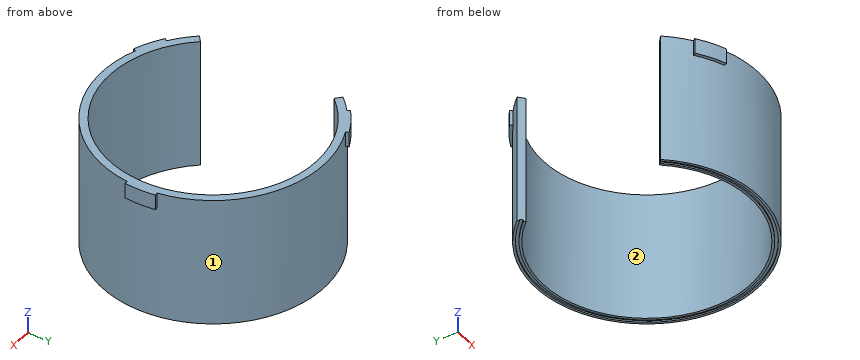
```python
from build123d import *

# Parameters (mm, degrees)
F3_DEPTH = 10
F5_DEPTH = 85


with BuildPart() as f1:
    # F0 (on Front) → F1 (revolve)
    with BuildSketch(Plane.XZ):
        Polygon((-68, 0), (-73, 0), (-73, -85), (-71.5, -85), (-71.5, -84), (-69.5, -84), (-69.5, -85), (-68, -85), align=None)
    revolve(axis=Axis((0, 0, -12.456594), (0, 0, -1)))

    # F2 (on face) → F3 (join)
    with BuildSketch(Plane.XY):
        with BuildLine():
            Line((-25.651511, -70.476947), (-24.96747, -68.597561))
            ThreePointArc((-24.96747, -68.597561), (-33.707649, -64.751791), (-41.87108, -59.798099))
            Line((-41.87108, -59.798099), (-43.018233, -61.436403))
            ThreePointArc((-43.018233, -61.436403), (-34.631146, -66.525812), (-25.651511, -70.476947))
        make_face()
        with BuildLine():
            Line((73.860581, 13.023613), (71.890966, 12.676317))
            ThreePointArc((71.890966, 12.676317), (72.93052, 3.184215), (72.722213, -6.362369))
            Line((72.722213, -6.362369), (74.714602, -6.536681))
            ThreePointArc((74.714602, -6.536681), (74.928617, 3.271454), (73.860581, 13.023613))
        make_face()
        with BuildLine():
            Line((-48.209071, 57.453333), (-46.923496, 55.921244))
            ThreePointArc((-46.923496, 55.921244), (-39.222871, 61.567576), (-30.851133, 66.160468))
            Line((-30.851133, 66.160468), (-31.69637, 67.973084))
            ThreePointArc((-31.69637, 67.973084), (-40.297471, 63.254358), (-48.209071, 57.453333))
        make_face()
    extrude(amount=-F3_DEPTH)

    # F4 (on face) → F5 (cut, through all)
    with BuildSketch(Plane.XY):
        with BuildLine():
            ThreePointArc((-55.509635, 47.409708), (-73, 0), (-55.509635, -47.409708))
            Line((-55.509635, -47.409708), (-51.707606, -44.162467))
            ThreePointArc((-51.707606, -44.162467), (-68, 0), (-51.707606, 44.162467))
            Line((-51.707606, 44.162467), (-55.509635, 47.409708))
        make_face()
    extrude(amount=-F5_DEPTH, mode=Mode.SUBTRACT)


solid = f1.part
```
For this review, take the finished solid that the model builds, in its own axes (mm). Face numbers are marked on the shaded views. A direction names the side the tool comes from. Give positions to 0.01 mm unless a question says otherwise; leave off trailing zeros. Write each loop counter-clockwise with the first axis right and the second up, starting at its lowest first coordinate (ties: lowest second). Pieces come first, ordered by that corner, then holes. Notation, with made-up numbers: M -24,89.25 L -9,89.25 A12 cw -9,95.25 Z; hole C -11,6 d5. An arc over 180 degrees is marked long. One line per item, written item: value.
1) Take a section at C-C, the plane y = 52. Write out the cut boundary in (x, z).
Results are:
outline: M -51.23,-85 L -49.07,-85 L -49.07,-84 L -46.11,-84 L -46.11,-85 L -43.82,-85 L -43.82,0 L -51.23,0 Z; M 43.82,-85 L 46.11,-85 L 46.11,-84 L 49.07,-84 L 49.07,-85 L 51.23,-85 L 51.23,0 L 43.82,0 Z
2) Take a section at D-D, the plane z = -35.5. Write out the cut boundary in (x, y), then the cut area to 3 significant figures.
Results are:
outline: M -55.51,-47.41 A73 ccw long -55.51,47.41 L -51.71,44.16 A68 cw long -51.71,-44.16 Z
area: 1,720 mm²
3) For the marked faces 1 and 2, list the 3-axis set-ups (+Z, -Z, +X, -X, +Y, -Y) from which the entire face can be reached by the end or side of a thin tool; tool diameter is ignored.
Results are:
face 1: -Z
face 2: +Z, -Z
4) For P1, Ø3, axis at x = -20, z = -34.5, coming from the +Y side; P2, Ø12, axis at x = 18, z = -44.5, coming from the +Y side; P3, Ø12, axis at x = 27.5, z = -75.5, coming from the +Y side, all flat-tipped, find the tip position at first contact; note any pin that passes through.
Results are:
P1: stops at y = 70.62
P2: stops at y = 72.01
P3: stops at y = 69.76
5) Take a section at A-A, the plane x = 0. Write out the cut boundary in (y, z).
Results are:
outline: M -73,-85 L -71.5,-85 L -71.5,-84 L -69.5,-84 L -69.5,-85 L -68,-85 L -68,0 L -73,0 Z; M 68,-85 L 69.5,-85 L 69.5,-84 L 71.5,-84 L 71.5,-85 L 73,-85 L 73,0 L 68,0 Z
6) For line 1 (Y direction, x = 0, z = -84.4); line 2 (X direction, y = 0, z = -35); line 3 (Y direction, x = 41, z = -48), list the stretches that pass through material, from the lowest coordinate up. Write a range as from..to.
Results are:
line 1: y = -73..-71.5, -69.5..-68, 68..69.5, 71.5..73
line 2: x = 68..73
line 3: y = -60.4..-54.25, 54.25..60.4
7) Take a section at B-B, the plane y = 0. Write out the cut boundary in (x, z).
Results are:
outline: M 68,-85 L 69.5,-85 L 69.5,-84 L 71.5,-84 L 71.5,-85 L 73,-85 L 73,-10 L 75,-10 L 75,0 L 68,0 Z
